Here's how the part is built. I have some questions about the finished solid (model axes, mm). A direction names the side the tool comes from. Give positions to 0.01 mm unless a question says otherwise; leave off trailing zeros. Write each loop counter-clockwise with the first axis right and the second up, starting at its lowest first coordinate (ties: lowest second). Pieces come first, ordered by that corner, then holes. Notation, with made-up numbers: (-21.5, 14) - (18.5, 14) arc R30 ccw to (18.5, 46) - close; hole circle Ø7 at (-32, 63). An arc over 180 degrees is marked (long way). One line per item, written item: value. Start each with the question number.
1) Imagine slicing it at B-B on y = 0.6. Count the separate pieces of the cut face and the enclosed holes in it, plus the area to 3 significant figures.
2) Imagine slicing it at A-A on x = 5.5. Write out the boundary of the cut face in (y, z), plus the area to 3 significant figures.
3) Please list where these lines run through material, in increasing order: L1, parallel to X at y = 2.7, z = 11.5; L2, parallel to X at y = 2.5, z = -4; L3, parallel to Z at x = -83, y = 1.3. Write a range as [from, to].
4) I'm going to push a flat-ended pin straight in: P1, Ø1.8, axis at x = -83, z = 11.5, coming from the +Y side. Where does the tip first touch, or does it pass through?
5) On a 3-axis mill with a long thin cutter (end or side, diameter ignored), from which of +Z, -Z, +X, -X, +Y, -Y can I reach the whole of each face in a straight line? I mean faces 5 (the flat face through (-1, 4, 0)), 6 (the flat face through (-83.5, 2, 0)). Say none if no direction works.
6) We'd pull the mould along X, two halves only. Please class faces 1 (the flat face through (-1, 2, 32.25)), 2 (the cylindrical face through (84.487, 2.028, 11.305)), 3 (the flat face through (-90, 2, 0)), 4 (the flat face through (90, 2, 0)): +X half, -X half, draft (parallel to the pull), parting line (faces both ways), or undercut.
from build123d import *

# Parameters (mm, degrees)
CROQUIS1_W              = 180
CROQUIS1_H              = 64.5
SALIENTE_EXTRUIR1_DEPTH = 4
CROQUIS2_W              = 2.5
CROQUIS2_H              = 10
CORTAR_EXTRUIR1_DEPTH   = 4
MATRIZL1_COUNT          = 2
MATRIZL1_PITCH          = 169.5
CROQUIS3_W              = 15
CROQUIS3_H              = 2.5
CORTAR_EXTRUIR2_DEPTH   = 4
CORTAR_EXTRUIR3_DEPTH   = 4
MATRIZL2_COUNT          = 2
MATRIZL2_PITCH          = 170.52
MATRIZL2_COUNT_DIR2     = 2
MATRIZL2_PITCH_DIR2     = 55.1
CROQUIS5_R              = 1.5
CORTAR_EXTRUIR4_DEPTH   = 4


with BuildPart() as part:
    # Croquis1 → Saliente-Extruir1 (new body)
    with BuildSketch(Plane(origin=(0, 0, 0), x_dir=(1, 0, 0), z_dir=(0, 1, 0))):
        Rectangle(CROQUIS1_W, CROQUIS1_H)
    extrude(amount=SALIENTE_EXTRUIR1_DEPTH)

    # Croquis2 → Cortar-Extruir1 (cut)
    with BuildSketch(Plane(origin=(0, 4, 0), x_dir=(1, 0, 0), z_dir=(0, 1, 0))):
        with Locations((84.75, 0)):
            Rectangle(CROQUIS2_W, CROQUIS2_H)
    cortar_extruir1 = extrude(amount=-CORTAR_EXTRUIR1_DEPTH, mode=Mode.SUBTRACT)

    # MatrizL1: Cortar-Extruir1 ×2
    with Locations(*[(-i * MATRIZL1_PITCH, 0, 0) for i in range(1, MATRIZL1_COUNT)]):
        add(cortar_extruir1, mode=Mode.SUBTRACT)

    # Croquis3 → Cortar-Extruir2 (cut)
    with BuildSketch(Plane(origin=(0, 0, 0), x_dir=(1, 0, 0), z_dir=(0, 1, 0))):
        with Locations((0, 27)):
            Rectangle(CROQUIS3_W, CROQUIS3_H)
        with Locations((0, -27)):
            Rectangle(CROQUIS3_W, CROQUIS3_H)
    extrude(amount=CORTAR_EXTRUIR2_DEPTH, mode=Mode.SUBTRACT)

    # Croquis4 → Cortar-Extruir3 (cut)
    with BuildSketch(Plane(origin=(0, 4, 0), x_dir=(1, 0, 0), z_dir=(0, 1, 0))):
        Polygon((-82.719317631, 27.55), (-83.989488223, 29.75), (-86.529829408, 29.75), (-87.8, 27.55), (-86.529829408, 25.35), (-83.989488223, 25.35), align=None)
    cortar_extruir3 = extrude(amount=-CORTAR_EXTRUIR3_DEPTH, mode=Mode.SUBTRACT)

    # MatrizL2: Cortar-Extruir3 2 × 2
    with Locations(*[(i * MATRIZL2_PITCH, 0, j * MATRIZL2_PITCH_DIR2) for i in range(MATRIZL2_COUNT) for j in range(MATRIZL2_COUNT_DIR2) if (i, j) != (0, 0)]):
        add(cortar_extruir3, mode=Mode.SUBTRACT)

    # Croquis5 → Cortar-Extruir4 (cut)
    with BuildSketch(Plane(origin=(0, 4, 0), x_dir=(1, 0, 0), z_dir=(0, 1, 0))):
        with Locations(Location((-83, 11.5, 0), (0, 0, 270))):
            Circle(CROQUIS5_R)
        with Locations(Location((-83, -11.5, 0), (0, 0, 270))):
            Circle(CROQUIS5_R)
        with Locations(Location((83, -11.5, 0), (0, 0, 270))):
            Circle(CROQUIS5_R)
        with Locations(Location((83, 11.5, 0), (0, 0, 270))):
            Circle(CROQUIS5_R)
    extrude(amount=-CORTAR_EXTRUIR4_DEPTH, mode=Mode.SUBTRACT)


solid = part.part
Numbers:
1. separate pieces: 1
1. enclosed holes: 12
1. area: 11,400 mm^2
2. outline: (0, -32.25) - (4, -32.25) - (4, -28.25) - (0, -28.25) - close; (0, -25.75) - (4, -25.75) - (4, 25.75) - (0, 25.75) - close; (0, 28.25) - (4, 28.25) - (4, 32.25) - (0, 32.25) - close
2. area: 238 mm^2
3. L1: [-90, -84.5], [-81.5, 81.5], [84.5, 90]
3. L2: [-90, -86], [-83.5, 83.5], [86, 90]
3. L3: [-32.25, -28.04], [-27.06, -13], [-10, 10], [13, 27.06], [28.04, 32.25]
4. P1: through
5. face 5: +Z, -Z, +X, -X, +Y
5. face 6: +Y, -Y
6. face 1: draft
6. face 2: undercut
6. face 3: -X half
6. face 4: +X half
